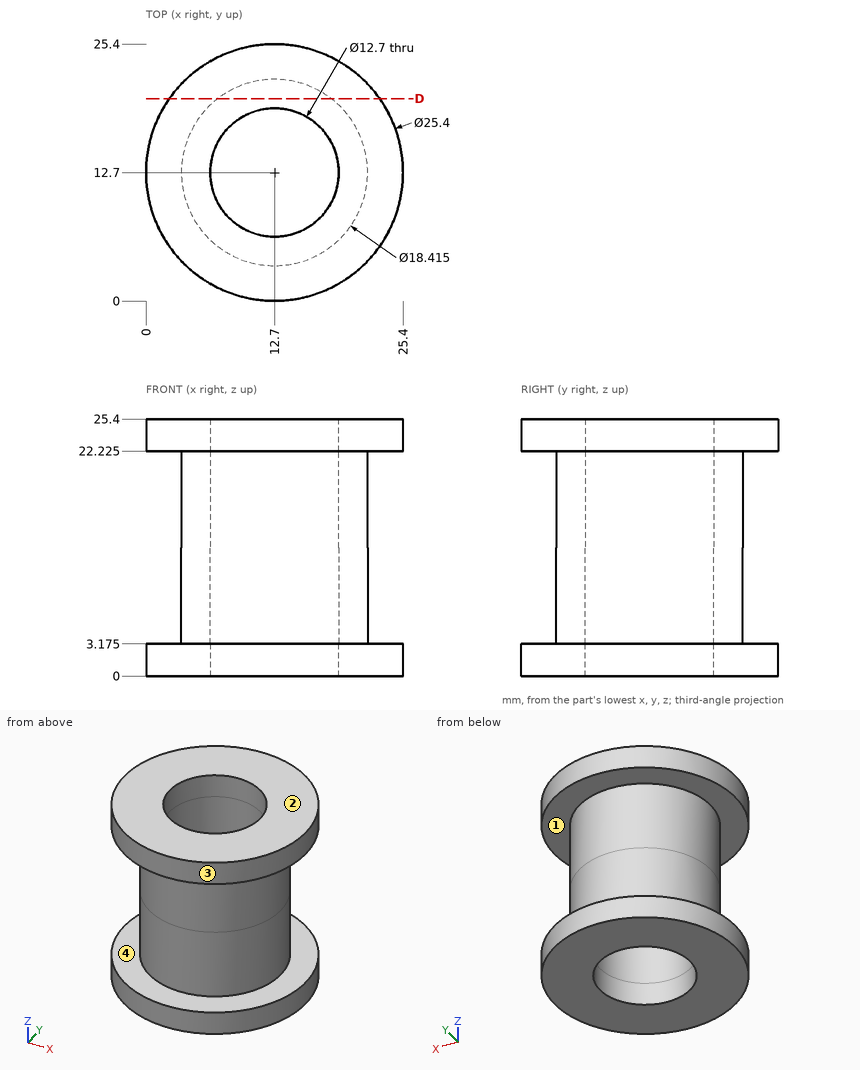
Source: three-view drawing plus pictorial views. Frame: mm from the lowest corner of the part. Give positions to 0.01 mm unless a question says otherwise; leave off trailing zeros. Loops run counter-clockwise (first coordinate to the right, second up) from the corner with the lowest first, then second, coordinate; pieces in that order, holes last.
1) Mould query, pull axis Z, two halves, no side actions, for the marked faces 1, 2, 3 and 4. Classes: released by +Z, released by -Z, zero draft, split by the parting line, or undercut.
A:
face 1: undercut
face 2: released by +Z
face 3: zero draft
face 4: undercut
2) Contact query for flat-ended pins moving along their axis: pin 1 (3 mm diameter, centred on x = 15.5, z = 4, fed in from -Y); pin 2 (4 mm diameter, centred on x = 3.5, z = 14, fed in from +Y); pin 3 (5 mm diameter, centred on x = 19.5, z = 22, fed in from +Y). Output: stop coordinate, or through.
A:
pin 1: stops at y = 0.09
pin 2: stops at y = 18.44
pin 3: stops at y = 24.65
3) Line query: L1, parallel to Y at x = 12.7, z = 23.6; L2, parallel to Z at x = 2, y = 18 (3 decimals); L3, parallel to X at y = 12.5, z = 12.5. Output: solid intervals per line, ascending.
A:
L1: y = 0 to 6.35, 19.05 to 25.4
L2: z = 0 to 3.175, 22.225 to 25.4
L3: x = 3.49 to 6.35, 19.05 to 21.91
4) Section query D-D on y = 20. Return the cut outline in (x, z) (3 decimals).
A:
outline: (2.308, 0) - (23.092, 0) - (23.092, 3.175) - (18.311, 3.175) - (18.311, 22.225) - (23.092, 22.225) - (23.092, 25.4) - (2.308, 25.4) - (2.308, 22.225) - (7.089, 22.225) - (7.089, 3.175) - (2.308, 3.175) - close
